Autodesk Inventor part; units mm, degrees
ref_plane "YZ Plane" through (0, 0, 0) normal (1, 0, 0) x (0, 1, 0)
ref_plane "XZ Plane" through (0, 0, 0) normal (0, 1, 0) x (-1, 0, 0)
ref_plane "XY Plane" through (0, 0, 0) normal (0, 0, 1) x (1, 0, 0)
sketch "Sketch1" plane through (0, 0, 0) normal (0, 0, 1) x (1, 0, 0)
  line L0 (-41.6667, 0) -> (41.6667, 0) construction
  line L1 (-41.6667, -8.3333) -> (41.6667, -8.3333)
  arc A0 (-41.6667, 8.3333) -> (-41.6667, -8.3333) centre (-41.6667, 0) ccw
  arc A1 (41.6667, -8.3333) -> (41.6667, 8.3333) centre (41.6667, 0) ccw
  line L2 (-8.75, 8.3333) -> (-41.6667, 8.3333)
  circle A2 centre (0, -4.1667) radius 2
  line L3 (0, 0) -> (-8.75, 0)
  line L4 (-8.75, 0) -> (-8.75, 8.3333)
  line L5 (0, 0) -> (8.75, 0)
  line L6 (8.75, 0) -> (8.75, 8.3333)
  line L7 (8.75, 8.3333) -> (41.6667, 8.3333)
  dimension "HL" = 41.6667
  dimension "d1" = 16.6667
  dimension "d10" = 4.1667
  dimension "HD" = 4
  dimension "d12" = 41.6667
  dimension "d13" = 8.75
  dimension "d14" = 8.75
  dimension "d17" = 8.75
  dimension "d18" = 8.3333
extrude "Main" add sketch "Sketch1" along normal blind 8.3333
sketch "Sketch2" plane through (-8.75, 0, 0) normal (1, 0, 0) x (0, 0, -1)
  line L0 (-8.3333, 8.3333) -> (-8.3333, 0)
  circle A0 centre (-8.3333, 4.1667) radius 2
  point P0 (0, 0)
  dimension "d19" = 4
extrude "Hole" cut sketch "Sketch2" along normal blind 42.5 and the other way blind 25
sketch "Sketch3" plane through (0, 0, 8.3333) normal (0, 0, 1) x (1, 0, 0)
  circle A0 centre (-41.6667, 0) radius 2
  line L0 (41.6667, 8.3333) -> (8.75, 8.3333)
  line L1 (-8.75, 8.3333) -> (-41.6667, 8.3333)
  point P0 (0, 0)
  dimension "d24" = 4
  dimension "d25" = 41.6667
  dimension "d29" = 8.3333
sketch "Sketch4" plane through (0, 0, 8.3333) normal (0, 0, 1) x (1, 0, 0)
  circle A0 centre (41.6667, 0) radius 2.4167
  line L0 (41.6667, 8.3333) -> (8.75, 8.3333)
  point P0 (0, 0)
  dimension "d30" = 41.6667
  dimension "d31" = 4.8333
  dimension "d32" = 8.3333
extrude "Pigg" add sketch "Sketch3" along normal blind 4.1667
extrude "Minuspigg" cut sketch "Sketch4" against normal blind 4.1667
sketch "Sketch5" plane through (0, 0, 8.3333) normal (0, 0, 1) x (1, 0, 0)
  point P0 (0, 0)
sketch "Sketch6" plane through (0, 0, 8.3333) normal (0, 0, 1) x (1, 0, 0)
  point P0 (0, 0)
sketch "Sketch7" plane through (0, 0, 8.3333) normal (0, 0, 1) x (1, 0, 0)
  point P0 (0, 0)
sketch "Sketch8" plane through (0, 0, 8.3333) normal (0, 0, 1) x (1, 0, 0)
  point P0 (0, 0)
sketch "Sketch9" plane through (0, 0, 8.3333) normal (0, 0, 1) x (1, 0, 0)
  point P0 (0, 0)
equation "\"d1\" = 0.4 * HL"
equation "\"d10\" = 0.1 * HL"
equation "\"d12\" = HL"
equation "\"d13\" = 0.2 * HL + Eps"
equation "\"d14\" = 0.2 * HL + Eps"
equation "\"d17\" = 0.2 * HL + Eps"
equation "\"d18\" = 0.2 * HL"
equation "\"d15\" = 0.2 * HL"
equation "\"d19\" = HD"
equation "\"d20\" = HL + 2 * Eps"
equation "\"d21\" = 0.6 * HL"
equation "\"d24\" = HD"
equation "\"d29\" = 0.2 * HL"
equation "\"d31\" = HD + 2 * Eps"
equation "\"d32\" = 0.2 * HL"
equation "\"d33\" = 0.1 * HL"
equation "\"d35\" = 0.1 * HL"
equation "\"Eps\" = 0.41667"
properties part number "1fjärdedel"
Read the model definition and answer for the solid it produces. Units are mm, in the model's axes. A direction names the side the tool comes from. Round coordinates to 2 decimals unless told otherwise and drop trailing zeros. Write each loop counter-clockwise with the first axis right and the second up, starting at its lowest first coordinate (ties: lowest second). Pieces come first, ordered by that corner, then holes.
1. The part is cut by section A-A, the plane x = 0. Determine the outline of the cut face in (y, z), then the cut area to 3 significant figures.
2. Given pin 1 Ø5 at (x, y) = (-36.5, 0.5) entering from +Z; pin 2 Ø4.5 at (x, y) = (41.67, 0) entering from +Z; pin 3 Ø2.5 at (y, z) = (4, 3.5) entering from +X, each flat-ended and moving along its own axis, determine where each tip first touches the part or whether it passes through.
3. Which of the six approach directions +Z, -Z, +X, -X, +Y, -Y give full straight-line access (tool end or side, diameter ignored) to faces 1 (the face through (39.252, 0.106, 6.279)), 2 (the face through (8.75, 4, 4)), 3 (the face through (50, 0, 4))?
4. The part is cut by section B-B, the plane y = 7.25. Determine the outline of the cut face in (x, z), then the cut area to 3 significant figures.
5. Determine the mould class of faces 4 (the face through (-25, 8.333, 4)), 5 (the face through (-50, 0, 4)), 6 (the face through (-33.75, 4, 8)) for opening direction X: pulls with the +X half, pulls with the -X half, needs draft (parallel to the pull), parting line crosses it, or undercut.
6. The part is cut by section D-D, the plane x = 21. Determine the outline of the cut face in (y, z), then the cut area to 3 significant figures.
7. The part is cut by section C-C, the plane z = 1.25. Determine the outline of the cut face in (x, y), then the cut area to 3 significant figures.
8. Straight lines are drawn through the part: L1, parallel to Y at x = 0, z = 3.5; L2, parallel to Z at x = 19.5, y = -6.75; L3, parallel to X at y = 5, z = 6. For each, find the intervals that lie inside material, in ascending order.
Values:
1. outline: (-8.33, 0) - (-6.17, 0) - (-6.17, 8.33) - (-8.33, 8.33) - close; (-2.17, 0) - (0, 0) - (0, 8.33) - (-2.17, 8.33) - close
1. area: 36.1 mm2
2. pin 1: stops at z = 8.33
2. pin 2: stops at z = 4.17
2. pin 3: stops at x = 49.53
3. face 1: +Z
3. face 2: +Z, -Z, +Y
3. face 3: +Z, -Z, +X
4. outline: (-45.78, 0) - (-8.75, 0) - (-8.75, 8.33) - (-45.78, 8.33) - close; (8.75, 0) - (45.78, 0) - (45.78, 8.33) - (8.75, 8.33) - close
4. area: 617 mm2
5. face 4: needs draft
5. face 5: pulls with the -X half
5. face 6: undercut
6. outline: (-8.33, 0) - (8.33, 0) - (8.33, 8.33) - (6.17, 8.33) arc R2 cw to (2.17, 8.33) - (-8.33, 8.33) - close
6. area: 133 mm2
7. outline: (-41.67, -8.33) - (41.67, -8.33) arc R8.33 ccw to (41.67, 8.33) - (8.75, 8.33) - (8.75, 0) - (-8.75, 0) - (-8.75, 8.33) - (-41.67, 8.33) arc R8.33 ccw to start; hole circle Ø4 at (0, -4.17)
7. area: 1,450 mm2
8. L1: y = -8.33 to -6.17, -2.17 to 0
8. L2: z = 0 to 8.33
8. L3: x = -48.33 to -8.75, 8.75 to 48.33
